from build123d import *

# Parameters (mm, degrees)
F1_DEPTH = 63.5
F0_W     = 20.1374943917
F0_H     = 19.05
F2_DEPTH = 50.8
F3_DEPTH = 7.9375
F5_R     = 6.35


with BuildPart() as f1:
    # F0 (on Front) → F1 (new body, symmetric)
    with BuildSketch(Plane.XZ):
        Polygon((-41.275, 9.525), (-41.275, -9.525), (41.275, -9.525), (41.275, 9.525), (22.225, 9.525), align=None)
    extrude(amount=F1_DEPTH, both=True)

    # F0 (on Front) → F2 (join)
    with BuildSketch(Plane.XZ):
        with BuildLine():
            Line((22.225, 9.525), (41.275, 9.525))
            Line((41.275, 9.525), (41.275, 27.0002))
            ThreePointArc((41.275, 27.0002), (45.9246798487, 38.2255201513), (57.15, 42.8752))
            Line((57.15, 42.8752), (60.325, 42.8752))
            Line((60.325, 42.8752), (60.325, 61.9252))
            Line((60.325, 61.9252), (57.15, 61.9252))
            add(Edge.make_bspline(
                [(54.9027937698, 61.8528281528), (55.6532384905, 61.8850370345), (56.4023888872, 61.9092238899), (57.15, 61.9252)],
                knots=[109.6972732661, 109.6972732661, 109.6972732661, 109.6972732661, 111.5045361635, 111.5045361635, 111.5045361635, 111.5045361635], degree=3))
            ThreePointArc((54.9027937698, 61.8528281528), (31.6721733404, 50.8881880631), (22.225, 27.0002))
            Line((22.225, 27.0002), (22.225, 9.525))
        make_face()
        with Locations((70.3937471959, 52.4002)):
            Rectangle(F0_W, F0_H)
    extrude(amount=F2_DEPTH)

    # F0 (on Front) → F3 (join, symmetric)
    with BuildSketch(Plane.XZ):
        with BuildLine():
            add(Edge.make_bspline(
                [(-41.275, 9.525), (-40.9668306676, 28.3876541447), (9.352287687, 59.8978129225), (54.9027937698, 61.8528281528)],
                knots=[0, 0, 0, 0, 109.6972732661, 109.6972732661, 109.6972732661, 109.6972732661], degree=3))
            Line((-41.275, 9.525), (22.225, 9.525))
            Line((22.225, 9.525), (22.225, 27.0002))
            ThreePointArc((22.225, 27.0002), (31.6721733404, 50.8881880631), (54.9027937698, 61.8528281528))
        make_face()
    extrude(amount=F3_DEPTH, both=True)

    # F0 (on Front) → F4 (revolve)
    with BuildSketch(Plane.XZ):
        Polygon((80.4624943917, 66.675), (80.4624943917, 61.9252), (80.4624943917, 42.8752), (80.4624943917, 38.1), (111.125, 38.1), (111.125, 66.675), align=None)
    revolve(axis=Axis((80.4624943917, 0, 52.3875), (0, 0, 1)))

    # F5
    f5_edges = [f1.edges().sort_by_distance(p)[0] for p in [
        (41.275, -63.5, 0),
        (-41.275, -63.5, 0),
        (41.275, 63.5, 0),
        (-41.275, 63.5, 0),
    ]]
    fillet(f5_edges, radius=F5_R)


solid = f1.part
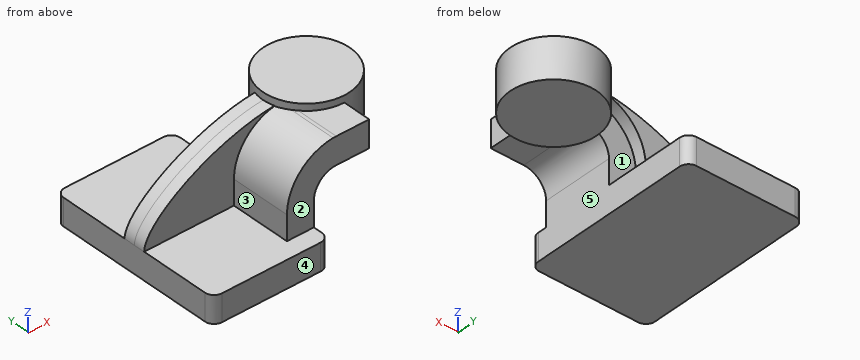
Can you work these out from the model? Positions are in its coordinate system, mm. Face numbers are marked on the shaded views. A direction names the side the tool comes from. Give positions to 0.01 mm unless a question says otherwise; leave off trailing zeros. Order: outer loops, then holes, each group sorted by start corner. A loop starts at its lowest first (then second) coordinate and runs counter-clockwise, first axis right, second up. Notation, with made-up numbers: M 82.5,69.25 L 126.5,69.25 A5 cw 126.5,76.25 Z; hole C 24,39 d10. An arc over 180 degrees is marked long. Use one line per item in the form item = value.
Item 1: If we section it at A-A, the plane y = 19: Write out the boundary of the cut face in (x, z) (3 decimals).
Values follow:
outline = M -41.275,-9.525 L 41.275,-9.525 L 41.275,9.525 L -41.275,9.525 Z; M 56.396,38.1 L 104.529,38.1 L 104.529,66.675 L 56.396,66.675 Z
Item 2: If we section it at B-B, the plane x = 77: Write out the boundary of the cut face in (y, z) (3 decimals), and give its area (3 significant figures).
Values follow:
outline = M -50.8,42.875 L -30.466,42.875 L -30.466,38.1 L 30.466,38.1 L 30.466,66.675 L -30.466,66.675 L -30.466,61.925 L -50.8,61.925 Z
area = 2,130 mm^2
Item 3: If we section it at D-D, the plane x = 101: Write out the boundary of the cut face in (y, z) (3 decimals).
Values follow:
outline = M -22.768,38.1 L 22.768,38.1 L 22.768,66.675 L -22.768,66.675 Z
Item 4: For the marked faces 1, 2, 3, 4 and 5, which set-ups out of +Z, -Z, +X, -X, +Y, -Y let a thin tool reach every point of the face, with its end or its side?
Values follow:
face_1 = +Y
face_2 = +Z, +X, -X, -Y
face_3 = +Z, -X, -Y
face_4 = +Z, -Z, +X, -X, -Y
face_5 = -Z, +X, +Y, -Y
Item 5: Will these pins go through, and if not, where does the flat tip stop? pin 1 Ø18.5 at (x, y) = (65.5, -11) entering from -Z; pin 2 Ø15.5 at (x, z) = (23.5, 45) entering from +Y; pin 3 Ø19 at (y, z) = (-32, 20) entering from -X (3 decimals).
Values follow:
pin_1 = 38.1
pin_2 = 7.94
pin_3 = 22.225
Item 6: If I drill on line 1 along X through (y, z) = (26, 2) (3 decimals); line 2 along Z through (x, y) = (75, -25) (3 decimals); line 3 along Y through (x, z) = (9, 38), over which ranges is the centre line in solid material (lowest first)? Write a range as [from, to].
Values follow:
line_1 = [-41.275, 41.275]
line_2 = [38.1, 66.675]
line_3 = [-7.94, 7.94]
Item 7: If we section it at C-C, the plane y = 32.5: Write out the boundary of the cut face in (x, z) (3 decimals).
Values follow:
outline = M -41.275,-9.525 L 41.275,-9.525 L 41.275,9.525 L -41.275,9.525 Z
